```python
from build123d import *

# Parameters (mm, degrees)
F0_W     = 6.604
F0_H     = 12.7
F0_R     = 3.175
F1_DEPTH = 8.89
F2_DEPTH = 6.35
F3_R     = 0.9525
F4_DEPTH = 12.7
F4_TAPER = -3
F5_R     = 1.27
F6_W     = 1.27
F6_H     = 0.762
F7_DEPTH = 6.35
F8_R     = 0.508


with BuildPart() as f1:
    # F0 (on Front) → F1 (new body)
    with BuildSketch(Plane.XZ):
        Rectangle(F0_W, F0_H)
        Circle(F0_R, mode=Mode.SUBTRACT)
        Circle(F0_R)
    extrude(amount=-F1_DEPTH)

    # F0 (on Front) → F2 (join)
    with BuildSketch(Plane.XZ):
        Circle(F0_R)
    extrude(amount=F2_DEPTH)

    # F3 (on face) → F4 (join)
    with BuildSketch(Plane.XZ.offset(6.35)):
        Circle(F3_R)
    extrude(amount=F4_DEPTH, taper=F4_TAPER)

    # F5
    f5_edges = [f1.edges().sort_by_distance(p)[0] for p in [
        (-1.618079, -19.05, 0),
    ]]
    fillet(f5_edges, radius=F5_R)

    # F6 (on face) → F7 (join)
    with BuildSketch(Plane(origin=(0, 8.89, 0), x_dir=(-1, 0, 0), z_dir=(0, 1, 0))):
        with Locations((0, 4.699)):
            Rectangle(F6_W, F6_H)
        Rectangle(F6_W, F6_H)
        with Locations((0, -4.699)):
            Rectangle(F6_W, F6_H)
    extrude(amount=F7_DEPTH)

    # F8
    f8_edges = [f1.edges().sort_by_distance(p)[0] for p in [
        (0.635, 15.24, 4.699),
        (-0.635, 15.24, 4.699),
        (0.635, 15.24, 0),
        (-0.635, 15.24, 0),
        (0.635, 15.24, -4.699),
        (-0.635, 15.24, -4.699),
    ]]
    fillet(f8_edges, radius=F8_R)


solid = f1.part
```
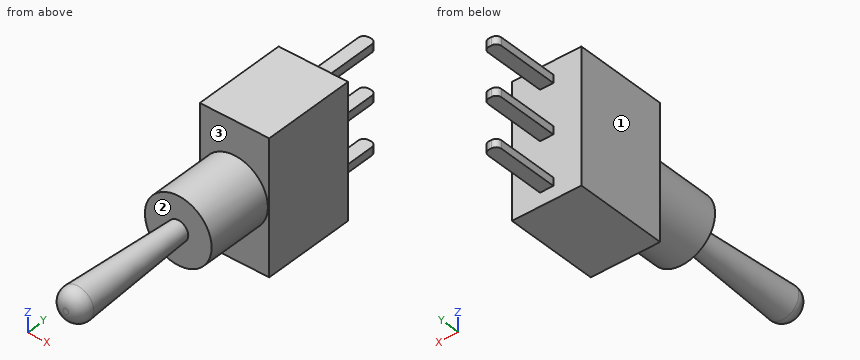
CAD build for the part. Positions are in the model's coordinates, mm. Face numbers are marked on the shaded views. A direction names the side the tool comes from. Round coordinates to 2 decimals unless told otherwise and drop trailing zeros. Order: outer loops, then holes, each group sorted by start corner. A loop starts at its lowest first (then second) coordinate and runs counter-clockwise, first axis right, second up.
Item 1: Saw through at B-B on z = 4.75. Write the cut outline in (x, y) (3 decimals).
Item 2: Saw through at D-D on y = -4. Write the cut outline in (x, z) (3 decimals).
Item 3: Pin check, flat tips, straight feed: pin 1 (0.6 mm diameter, centred on y = 11, z = 4.5, fed in from -X) (3 decimals); pin 2 (2 mm diameter, centred on x = -1.5, z = 0, fed in from +Y); pin 3 (4 mm diameter, centred on y = -6, z = 3, fed in from +X). Stop position of each tip, or through.
Item 4: Probe line 1 along Y through (x, z) = (2, 5.25); line 2 along X through (y, z) = (10, -4.5) (3 decimals); line 3 along Y through (x, z) = (2, -2). List the from-to ranges inside material, lowest first.
Item 5: Saw through at A-A on y = 9.5. Write the cut outline in (x, z) (3 decimals), then the cut area to 3 significant figures.
Item 6: Saw through at C-C on x = -2.5. Write the cut outline in (y, z), then the cut area to 3 significant figures.
Item 7: Tool access for the marked faces 1, 2 and 3: list every direction of +Z, -Z, +X, -X, +Y, -Y with a clear straight run to the whole face (end or side of a thin tool).
Reported:
1. outline: (-3.302, 0) - (3.302, 0) - (3.302, 8.89) - (0.635, 8.89) - (0.635, 14.732) arc R0.508 ccw to (0.127, 15.24) - (-0.127, 15.24) arc R0.508 ccw to (-0.635, 14.732) - (-0.635, 8.89) - (-3.302, 8.89) - close
2. outline: circle Ø6.35 at (0, 0)
3. pin 1: stops at x = -0.635
3. pin 2: stops at y = 15.08
3. pin 3: stops at x = 3.01
4. line 1: y = 0 to 8.89
4. line 2: x = -0.635 to 0.635
4. line 3: y = -6.35 to 8.89
5. outline: (-0.635, -5.08) - (0.635, -5.08) - (0.635, -4.318) - (-0.635, -4.318) - close; (-0.635, -0.381) - (0.635, -0.381) - (0.635, 0.381) - (-0.635, 0.381) - close; (-0.635, 4.318) - (0.635, 4.318) - (0.635, 5.08) - (-0.635, 5.08) - close
5. area: 2.90 mm2
6. outline: (-6.35, -1.96) - (0, -1.96) - (0, -6.35) - (8.89, -6.35) - (8.89, 6.35) - (0, 6.35) - (0, 1.96) - (-6.35, 1.96) - close
6. area: 138 mm2
7. face 1: +Z, -Z, -X, +Y, -Y
7. face 2: none
7. face 3: -Y
